The listing builds one solid part. Answer for the finished solid, in the listing's coordinates (mm). Face numbers are marked on the shaded views. A direction names the side the tool comes from. Give positions to 0.01 mm unless a question says otherwise; leave off trailing zeros. Loops run counter-clockwise (first coordinate to the right, second up) from the corner with the lowest first, then second, coordinate; pieces in that order, holes last. Notation, with made-up numbers: M 30.25,-3.5 L 76.25,-3.5 A19 ccw 76.25,2.5 Z; hole C 62,36.25 d2. An arc over 180 degrees is marked long. One line per item, written item: value. Start each with the question number.
Q1. A cutting plane is placed at C-C, the plane z = 7.5. Determine the outline of the cut face in (x, y).
Q2. A cutting plane is placed at A-A, the plane z = 13.5. Determine the outline of the cut face in (x, y).
Q3. The mould has two halves that part along X. Classify the marked faces 3, 4, 5 and 6: +X half, -X half, draft (parallel to the pull), parting line (faces both ways), or undercut.
Q4. Consider L1, parallel to Z at x = -15.35, y = -10; L2, parallel to X at y = -6.25, z = 9; L3, parallel to X at y = -11.5, z = 6.75. Determine where each line is inside the solid, lowest interval first.
Q5. A cutting plane is placed at D-D, the plane y = -15.5. Determine the outline of the cut face in (x, z), and give its area (3 significant figures).
Q6. For the marked faces 1 and 2, determine the directions among +Z, -Z, +X, -X, +Y, -Y from which every point of the face is accessible in a straight line to the end or side of a thin tool.
Q7. A cutting plane is placed at B-B, the plane y = -10. Determine the outline of the cut face in (x, z), and give its area (3 significant figures).
Q8. Flat-ended cylindrical pins translate along their axes: pin 1 (4 mm diameter, centred on y = -10, z = 7.5, fed in from +X); pin 2 (2 mm diameter, centred on x = 5.5, y = -8.5, fed in from +Z); pin 3 (3 mm diameter, centred on y = -9.5, z = 7.5, fed in from -X); pin 4 (1.5 mm diameter, centred on y = -10, z = 7.5, fed in from +X). Find the tip coordinate at first contact, or state that the pin passes through.
from build123d import *

# Parameters (mm, degrees)
PAD_DEPTH       = 20
SKETCH001_R     = 1.25
POCKET_DEPTH    = 46.001
SKETCH002_R     = 2.5
POCKET001_DEPTH = 3
SKETCH003_R     = 2.5
POCKET002_DEPTH = 3


with BuildPart() as part:
    # Sketch (on XZ_Plane of Origin) → Pad (new body)
    with BuildSketch(Plane.XZ):
        Polygon((-19.90873, 15), (-19.90873, 0), (26.09127, 0), (26.09127, 15), (21.09127, 15), (21.09127, 5), (-14.90873, 5), (-14.90873, 15), align=None)
    extrude(amount=PAD_DEPTH)

    # Sketch001 (on Face3 of Pad) → Pocket (cut, through all)
    with BuildSketch(Plane.YZ.offset(26.09127)):
        with Locations((-10, 7.5)):
            Circle(SKETCH001_R)
    extrude(amount=-POCKET_DEPTH, mode=Mode.SUBTRACT)

    # Sketch002 (on Face1 of Pocket) → Pocket001 (cut)
    with BuildSketch(Plane(origin=(-19.90873, 0, 0), x_dir=(0, -1, 0), z_dir=(-1, 0, 0))):
        with Locations((10, 7.5)):
            Circle(SKETCH002_R)
    extrude(amount=-POCKET001_DEPTH, mode=Mode.SUBTRACT)

    # Sketch003 (on Face8 of Pocket001) → Pocket002 (cut)
    with BuildSketch(Plane.YZ.offset(26.09127)):
        with Locations((-10, 7.5)):
            Circle(SKETCH003_R)
    extrude(amount=-POCKET002_DEPTH, mode=Mode.SUBTRACT)


solid = part.part
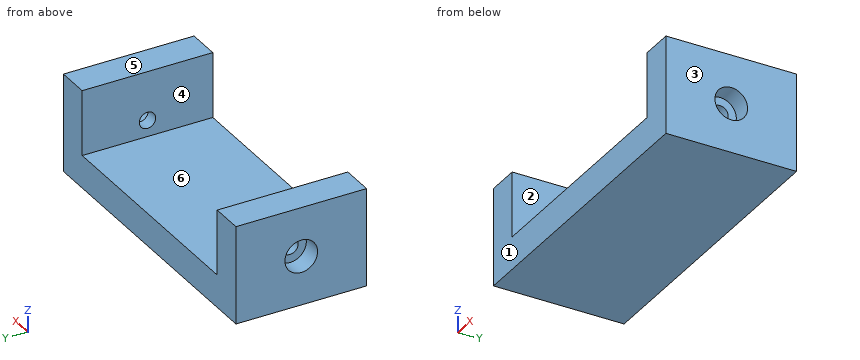
Answer block:
1. outline: M -19.91,-20 L -14.91,-20 L -14.91,-11.25 L -16.91,-11.25 L -16.91,-12.5 L -19.91,-12.5 Z; M -19.91,-7.5 L -16.91,-7.5 L -16.91,-8.75 L -14.91,-8.75 L -14.91,0 L -19.91,0 Z; M 21.09,-20 L 26.09,-20 L 26.09,-12.5 L 23.09,-12.5 L 23.09,-11.25 L 21.09,-11.25 Z; M 21.09,-8.75 L 23.09,-8.75 L 23.09,-7.5 L 26.09,-7.5 L 26.09,0 L 21.09,0 Z
2. outline: M -19.91,-20 L -14.91,-20 L -14.91,0 L -19.91,0 Z; M 21.09,-20 L 26.09,-20 L 26.09,0 L 21.09,0 Z
3. face 3: +X half
3. face 4: undercut
3. face 5: draft
3. face 6: undercut
4. L1: 0 to 6.25, 8.75 to 15
4. L2: -19.91 to -14.91, 21.09 to 26.09
4. L3: -16.91 to -14.91, 21.09 to 23.09
5. outline: M -19.91,0 L 26.09,0 L 26.09,15 L 21.09,15 L 21.09,5 L -14.91,5 L -14.91,15 L -19.91,15 Z
5. area: 330 mm^2
6. face 1: +Z, -Z, +X, -X, -Y
6. face 2: +Z, +Y, -Y
7. outline: M -19.91,0 L 26.09,0 L 26.09,5 L 23.09,5 L 23.09,6.25 L 21.09,6.25 L 21.09,5 L -14.91,5 L -14.91,6.25 L -16.91,6.25 L -16.91,5 L -19.91,5 Z; M -19.91,10 L -16.91,10 L -16.91,8.75 L -14.91,8.75 L -14.91,15 L -19.91,15 Z; M 21.09,8.75 L 23.09,8.75 L 23.09,10 L 26.09,10 L 26.09,15 L 21.09,15 Z
7. area: 290 mm^2
8. pin 1: x = 23.09
8. pin 2: z = 5
8. pin 3: x = -16.91
8. pin 4: through
